Read the model definition and answer for the solid it produces. Units are mm, in the model's axes. Face numbers are marked on the shaded views. A direction names the side the tool comes from. Round coordinates to 2 decimals unless told otherwise and drop trailing zeros. Loops run counter-clockwise (first coordinate to the right, second up) from the corner with the lowest first, then second, coordinate; pieces in that order, holes last. Notation, with made-up numbers: M -35,23 L -4,23 A32 ccw -4,52 Z; hole C -14.5,50.5 d11. An arc over 180 degrees is marked long. Answer as CSV lines item,"result".
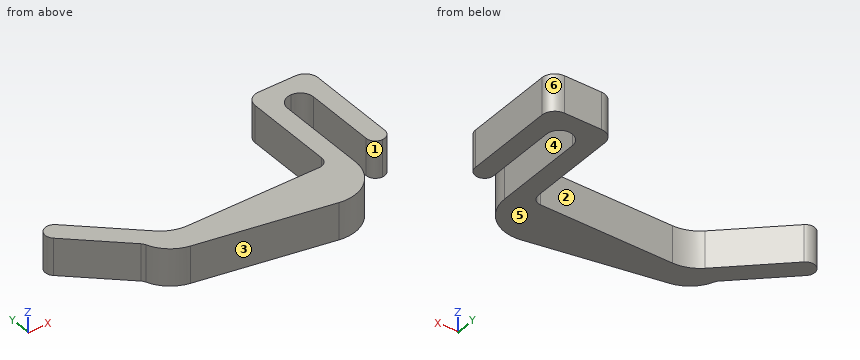
```python
from build123d import *

# Parameters (mm, degrees)
F1_DEPTH = 10
F2_R     = 3.49999
F3_R     = 2.49999
F4_R     = 10


# Not quite as in the source:
# - a fillet or chamfer is up to 0.001 mm smaller than in the source, because OpenCascade refuses the exact size


with BuildPart() as f1:
    # F0 (on Top) → F1 (new body)
    with BuildSketch(Plane.XY):
        Polygon((5, -15), (5, 0), (5, 25), (12, 25), (12, 0), (17, 0), (17, 30), (0, 30), (0, 0), (-42, 0), (-49.3313959282, 0), (-49.3313959282, -5), align=None)
        Polygon((-65.8878954456, 15.4391855737), (-49.3313959282, 0), (-42, 0), (-62.4779036453, 19.0959540817), align=None)
    extrude(amount=F1_DEPTH)

    # F2 (radius 3.5 in the source; OpenCascade refuses exactly that, so slightly less here)
    f2_edges = [f1.edges().sort_by_distance(p)[0] for p in [
        (5, 25, 5),
        (12, 25, 5),
        (0, 30, 5),
        (17, 30, 5),
    ]]
    fillet(f2_edges, radius=F2_R)

    # F3 (radius 2.5 in the source; OpenCascade refuses exactly that, so slightly less here)
    f3_edges = [f1.edges().sort_by_distance(p)[0] for p in [
        (0, 0, 5),
        (17, 0, 5),
        (12, 0, 5),
        (-49.331396, 0, 5),
        (-62.477904, 19.095954, 5),
        (-65.887895, 15.439186, 5),
    ]]
    fillet(f3_edges, radius=F3_R)

    # F4
    f4_edges = [f1.edges().sort_by_distance(p)[0] for p in [
        (-2.49999, 0, 5),
        (5, -15, 5),
        (-49.331396, -5, 5),
        (-42, 0, 5),
    ]]
    fillet(f4_edges, radius=F4_R)


solid = f1.part
```
1) Find section D-D, the plane x = -20.5. Give the vertices of the cut face in (y, z).
Evaluation:
outline,"M -10.31,0 L 0,0 L 0,10 L -10.31,10 Z"
2) Straight lines are drawn through the part: line 1 (X direction, y = 3, z = 6.5); line 2 (X direction, y = 9, z = 1.5); line 3 (X direction, y = 20.5, z = 9.75). For each, find the intervals that lie inside material, in ascending order.
Evaluation:
line 1,"x = -52.55 to -45.22, 0 to 5, 12 to 17"
line 2,"x = -58.98 to -51.65, 0 to 5, 12 to 17"
line 3,"x = 0 to 5, 12 to 17"
3) Find section C-C, the plane x = -9.5. Give the vertices of the cut face in (y, z), then the cut area to 3 significant figures.
Evaluation:
outline,"M -12.33,0 L 0,0 L 0,10 L -12.33,10 Z"
area,"123 mm^2"
4) Determine the mould class of the marked faces 4, 5 and 6 for opening direction X: released by +X, released by -X, zero draft, split by the parting line, or undercut.
Evaluation:
face 4,"undercut"
face 5,"zero draft"
face 6,"released by +X"
5) Find section A-A, the plane y = 8.5. Give the vertices of the cut face in (x, z).
Evaluation:
outline,"M -58.45,0 L -51.12,0 L -51.12,10 L -58.45,10 Z; M 0,0 L 5,0 L 5,10 L 0,10 Z; M 12,0 L 17,0 L 17,10 L 12,10 Z"
6) Each of these flat-tipped pins is pushed along its axis until it touches: P1, Ø3, axis at y = 9.5, z = 3, coming from the -X side; P2, Ø1, axis at y = 0, z = 7, coming from the -X side; P3, Ø4, axis at x = -42.5, z = 3.5, coming from the +Y side. Where does it stop, or does it pass through?
Evaluation:
P1,"stops at x = -61.13"
P2,"stops at x = -49.9"
P3,"stops at y = 2.35"
7) A tool of negligible diameter and unlimited length cuts with its end or side. For the marked faces 1, 2 and 3, from which of +Z, -Z, +X, -X, +Y, -Y can it reach the whole face along a straight path? Write none if from no direction.
Evaluation:
face 1,"+Z, -Z, -Y"
face 2,"+Z, -Z, +Y"
face 3,"+Z, -Z, -X, -Y"
8) Find section B-B, the plane y = 16.5. Give the vertices of the cut face in (x, z).
Evaluation:
outline,"M -64.67,0 L -59.69,0 L -59.69,10 L -64.67,10 Z; M 0,0 L 5,0 L 5,10 L 0,10 Z; M 12,0 L 17,0 L 17,10 L 12,10 Z"
